```python
from build123d import *

# Parameters (mm, degrees)
F0_W     = 151.6
F0_H     = 151.6
F0_W_2   = 29.6
F0_H_2   = 0.4
F0_W_3   = 0.4
F0_H_3   = 29.6
F0_W_4   = 14.2
F0_H_4   = 14.2
F0_W_5   = 0.8
F0_H_5   = 0.8
F1_DEPTH = 0.2


with BuildPart() as f1:
    # F0 (on Top) → F1 (new body)
    with BuildSketch(Plane.XY):
        Rectangle(F0_W, F0_H)
        Polygon((75, -0.4), (75, -75), (0.4, -75), (0, -75), (-0.4, -75), (-75, -75), (-75, -0.4), (-75, 0), (-75, 0.4), (-75, 75), (-0.4, 75), (0, 75), (0.4, 75), (75, 75), (75, 0.4), (75, 0), align=None, mode=Mode.SUBTRACT)
        Polygon((-60.8, 60.8), (-60.8, 0.4), (-60, 0.4), (-60, 60), (-0.4, 60), (-0.4, 60.8), align=None)
        Polygon((0.4, -60), (0.4, -60.8), (60.8, -60.8), (60.8, -0.4), (60, -0.4), (60, -60), align=None)
        Polygon((-60.8, -60.8), (-0.4, -60.8), (-0.4, -60), (-60, -60), (-60, -0.4), (-60.8, -0.4), align=None)
        Polygon((60, 0.4), (60.8, 0.4), (60.8, 60.8), (0.4, 60.8), (0.4, 60), (60, 60), align=None)
        Polygon((-45.8, 45.8), (-45.8, 0.4), (-45, 0.4), (-45, 45), (-0.4, 45), (-0.4, 45.8), align=None)
        Polygon((45, 0.4), (45.8, 0.4), (45.8, 45.8), (0.4, 45.8), (0.4, 45), (45, 45), align=None)
        Polygon((-45.8, -45.8), (-0.4, -45.8), (-0.4, -45), (-45, -45), (-45, -0.4), (-45.8, -0.4), align=None)
        Polygon((0.4, -45), (0.4, -45.8), (45.8, -45.8), (45.8, -0.4), (45, -0.4), (45, -45), align=None)
        Polygon((-30.8, 30.8), (-30.8, 0.4), (-30, 0.4), (-30, 30), (-0.4, 30), (-0.4, 30.8), align=None)
        Polygon((-30.8, -30.8), (-0.4, -30.8), (-0.4, -30), (-30, -30), (-30, -0.4), (-30.8, -0.4), align=None)
        Polygon((30, 0.4), (30.8, 0.4), (30.8, 30.8), (0.4, 30.8), (0.4, 30), (30, 30), align=None)
        Polygon((0.4, -30), (0.4, -30.8), (30.8, -30.8), (30.8, -0.4), (30, -0.4), (30, -30), align=None)
        with Locations((15.2, 0.2)):
            Rectangle(F0_W_2, F0_H_2)
        with Locations((-15.2, 0.2)):
            Rectangle(F0_W_2, F0_H_2)
        with Locations((15.2, -0.2)):
            Rectangle(F0_W_2, F0_H_2)
        with Locations((-0.2, 15.2)):
            Rectangle(F0_W_3, F0_H_3)
        with Locations((-15.2, -0.2)):
            Rectangle(F0_W_2, F0_H_2)
        with Locations((-0.2, -15.2)):
            Rectangle(F0_W_3, F0_H_3)
        with Locations((0.2, -15.2)):
            Rectangle(F0_W_3, F0_H_3)
        with Locations((0.2, 15.2)):
            Rectangle(F0_W_3, F0_H_3)
        with Locations((-52.9, -0.2)):
            Rectangle(F0_W_4, F0_H_2)
        with Locations((52.9, -0.2)):
            Rectangle(F0_W_4, F0_H_2)
        with Locations((-37.9, -0.2)):
            Rectangle(F0_W_4, F0_H_2)
        with Locations((67.9, 0.2)):
            Rectangle(F0_W_4, F0_H_2)
        with Locations((-67.9, 0.2)):
            Rectangle(F0_W_4, F0_H_2)
        with Locations((-52.9, 0.2)):
            Rectangle(F0_W_4, F0_H_2)
        with Locations((37.9, 0.2)):
            Rectangle(F0_W_4, F0_H_2)
        with Locations((52.9, 0.2)):
            Rectangle(F0_W_4, F0_H_2)
        with Locations((-37.9, 0.2)):
            Rectangle(F0_W_4, F0_H_2)
        with Locations((0.2, -67.9)):
            Rectangle(F0_W_3, F0_H_4)
        with Locations((-67.9, -0.2)):
            Rectangle(F0_W_4, F0_H_2)
        with Locations((-0.2, 52.9)):
            Rectangle(F0_W_3, F0_H_4)
        with Locations((-0.2, -52.9)):
            Rectangle(F0_W_3, F0_H_4)
        with Locations((0.2, 67.9)):
            Rectangle(F0_W_3, F0_H_4)
        with Locations((67.9, -0.2)):
            Rectangle(F0_W_4, F0_H_2)
        with Locations((0.2, -37.9)):
            Rectangle(F0_W_3, F0_H_4)
        with Locations((0.2, 37.9)):
            Rectangle(F0_W_3, F0_H_4)
        with Locations((37.9, -0.2)):
            Rectangle(F0_W_4, F0_H_2)
        with Locations((0.2, 52.9)):
            Rectangle(F0_W_3, F0_H_4)
        with Locations((-0.2, 37.9)):
            Rectangle(F0_W_3, F0_H_4)
        with Locations((-0.2, -37.9)):
            Rectangle(F0_W_3, F0_H_4)
        with Locations((-0.2, -67.9)):
            Rectangle(F0_W_3, F0_H_4)
        with Locations((-0.2, 67.9)):
            Rectangle(F0_W_3, F0_H_4)
        with Locations((0.2, -52.9)):
            Rectangle(F0_W_3, F0_H_4)
        with Locations((-45.4, 0.2)):
            Rectangle(F0_W_5, F0_H_2)
        with Locations((-60.4, -0.2)):
            Rectangle(F0_W_5, F0_H_2)
        with Locations((30.4, -0.2)):
            Rectangle(F0_W_5, F0_H_2)
        with Locations((-60.4, 0.2)):
            Rectangle(F0_W_5, F0_H_2)
        with Locations((60.4, 0.2)):
            Rectangle(F0_W_5, F0_H_2)
        with Locations((45.4, 0.2)):
            Rectangle(F0_W_5, F0_H_2)
        with Locations((-45.4, -0.2)):
            Rectangle(F0_W_5, F0_H_2)
        with Locations((-30.4, -0.2)):
            Rectangle(F0_W_5, F0_H_2)
        with Locations((-0.2, 45.4)):
            Rectangle(F0_W_3, F0_H_5)
        with Locations((-0.2, -30.4)):
            Rectangle(F0_W_3, F0_H_5)
        with Locations((60.4, -0.2)):
            Rectangle(F0_W_5, F0_H_2)
        with Locations((0.2, 60.4)):
            Rectangle(F0_W_3, F0_H_5)
        with Locations((0.2, -60.4)):
            Rectangle(F0_W_3, F0_H_5)
        with Locations((-30.4, 0.2)):
            Rectangle(F0_W_5, F0_H_2)
        with Locations((30.4, 0.2)):
            Rectangle(F0_W_5, F0_H_2)
        with Locations((-0.2, -60.4)):
            Rectangle(F0_W_3, F0_H_5)
        with Locations((-0.2, 60.4)):
            Rectangle(F0_W_3, F0_H_5)
        with Locations((-0.2, -45.4)):
            Rectangle(F0_W_3, F0_H_5)
        with Locations((0.2, 30.4)):
            Rectangle(F0_W_3, F0_H_5)
        with Locations((0.2, -30.4)):
            Rectangle(F0_W_3, F0_H_5)
        with Locations((45.4, -0.2)):
            Rectangle(F0_W_5, F0_H_2)
        with Locations((0.2, -45.4)):
            Rectangle(F0_W_3, F0_H_5)
        with Locations((0.2, 45.4)):
            Rectangle(F0_W_3, F0_H_5)
        with Locations((-0.2, 30.4)):
            Rectangle(F0_W_3, F0_H_5)
        with Locations((-0.2, 0.2)):
            Rectangle(F0_W_3, F0_H_2)
        with Locations((-0.2, -0.2)):
            Rectangle(F0_W_3, F0_H_2)
        with Locations((0.2, 0.2)):
            Rectangle(F0_W_3, F0_H_2)
        with Locations((0.2, -0.2)):
            Rectangle(F0_W_3, F0_H_2)
    extrude(amount=F1_DEPTH)


solid = f1.part
```
The model under review builds one solid part; all positions refer to its coordinate system, in mm. Round coordinates to 2 decimals unless told otherwise and drop trailing zeros. Loops run counter-clockwise (first coordinate to the right, second up) from the corner with the lowest first, then second, coordinate; pieces in that order, holes last. Notation, with made-up numbers: (26.25, 2) - (76.25, 2) arc R20 ccw to (76.25, 35) - close; hole circle Ø6 at (-37, -35.5). An arc over 180 degrees is marked (long way). Write each question's results on one line, items separated by ' | '. Start each with the question number.
Q1. Wall thickness on line 1 along X through (y, z) = (-48, 0.15); line 2 along X through (y, z) = (61.5, 0.1): over which ranges is each line inside the solid? List them lowest first. Write a range as [from, to].
Q2. Take a section at C-C on x = 35. Give the boundary of the cut face in (y, z), plus the area to 3 significant figures.
Q3. Insertion check: P1, Ø2, axis at x = -48, y = -44, coming from the -Z side. The pin has a flat end and moves straight along its axis. Give the tip position at first contact, or say it passes through.
Q4. Take a section at D-D on z = 0.1. Give the number of separate pieces and of enclosed holes in the cut face, plus the area to 3 significant figures.
Q5. Take a section at A-A on x = -56. Give the boundary of the cut face in (y, z).
Data:
1) line 1: x = [-75.8, -75], [-60.8, -60], [-0.4, 0.4], [60, 60.8], [75, 75.8] | line 2: x = [-75.8, -75], [-0.4, 0.4], [75, 75.8]
2) outline: (-75.8, 0) - (-75, 0) - (-75, 0.2) - (-75.8, 0.2) - close; (-60.8, 0) - (-60, 0) - (-60, 0.2) - (-60.8, 0.2) - close; (-45.8, 0) - (-45, 0) - (-45, 0.2) - (-45.8, 0.2) - close; (-0.4, 0) - (0.4, 0) - (0.4, 0.2) - (-0.4, 0.2) - close; (45, 0) - (45.8, 0) - (45.8, 0.2) - (45, 0.2) - close; (60, 0) - (60.8, 0) - (60.8, 0.2) - (60, 0.2) - close; (75, 0) - (75.8, 0) - (75.8, 0.2) - (75, 0.2) - close | area: 1.12 mm²
3) P1: passes through
4) separate pieces: 1 | enclosed holes: 16 | area: 1,590 mm²
5) outline: (-75.8, 0) - (-75, 0) - (-75, 0.2) - (-75.8, 0.2) - close; (-60.8, 0) - (-60, 0) - (-60, 0.2) - (-60.8, 0.2) - close; (-0.4, 0) - (0.4, 0) - (0.4, 0.2) - (-0.4, 0.2) - close; (60, 0) - (60.8, 0) - (60.8, 0.2) - (60, 0.2) - close; (75, 0) - (75.8, 0) - (75.8, 0.2) - (75, 0.2) - close
